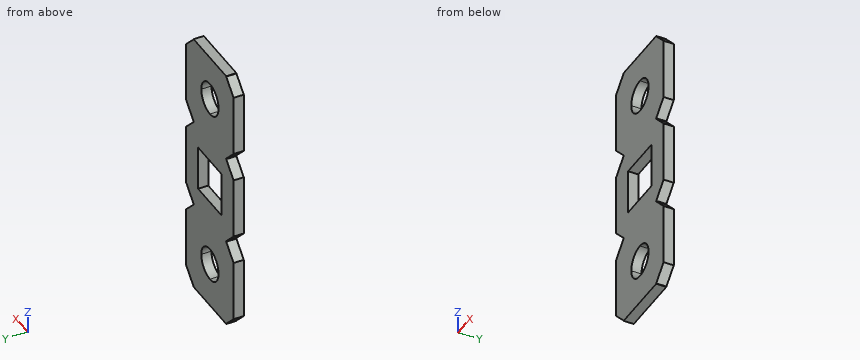
from build123d import *

# Parameters (mm, degrees)
STOCK_HS_LOCK_BAR_3_LONG_1_OUTLINE_W = 6.35
STOCK_HS_LOCK_BAR_3_LONG_1_OUTLINE_H = 6.35
STOCK_HS_LOCK_BAR_3_LONG_1_DEPTH     = 1.4224
BOSS_EXTRUDE1_START                  = -1.4224
BOSS_EXTRUDE1_DEPTH                  = 1.4224


# Read off the part's stored shape, not the designer's step: Stock-HS lock bar 3 long-1
with BuildPart() as part:
    # Stock-HS lock bar 3 long-1 outline → Stock-HS lock bar 3 long-1 (new body)
    with BuildSketch(Plane(origin=(0, 0, 0), x_dir=(1, 0, 0), z_dir=(0, 1, 0))):
        with BuildLine():
            Line((12.7, 36.073014945), (10.762817506, 38.010197439))
            ThreePointArc((10.762817506, 38.010197439), (10.725620068, 38.1), (10.762817506, 38.189802561))
            Line((10.762817506, 38.189802561), (12.7, 40.126985055))
            Line((12.7, 40.126985055), (12.7, 48.773014945))
            Line((12.7, 48.773014945), (10.762817506, 50.710197439))
            ThreePointArc((10.762817506, 50.710197439), (10.725620068, 50.8), (10.762817506, 50.889802561))
            Line((10.762817506, 50.889802561), (12.7, 52.826985055))
            Line((12.7, 52.826985055), (12.7, 61.473014945))
            Line((12.7, 61.473014945), (10.762817506, 63.410197439))
            ThreePointArc((10.762817506, 63.410197439), (10.735287367, 63.451399204), (10.725620068, 63.5))
            Line((10.725620068, 63.5), (1.974379932, 63.5))
            ThreePointArc((1.974379932, 63.5), (1.964712633, 63.451399204), (1.937182494, 63.410197439))
            Line((1.937182494, 63.410197439), (0, 61.473014945))
            Line((0, 61.473014945), (0, 52.826985055))
            Line((0, 52.826985055), (1.937182494, 50.889802561))
            ThreePointArc((1.937182494, 50.889802561), (1.974379932, 50.8), (1.937182494, 50.710197439))
            Line((1.937182494, 50.710197439), (0, 48.773014945))
            Line((0, 48.773014945), (0, 40.126985055))
            Line((0, 40.126985055), (1.937182494, 38.189802561))
            ThreePointArc((1.937182494, 38.189802561), (1.974379932, 38.1), (1.937182494, 38.010197439))
            Line((1.937182494, 38.010197439), (0, 36.073014945))
            Line((0, 36.073014945), (0, 27.426985055))
            Line((0, 27.426985055), (1.937182494, 25.489802561))
            ThreePointArc((1.937182494, 25.489802561), (1.964712633, 25.448600796), (1.974379932, 25.4))
            Line((1.974379932, 25.4), (10.725620068, 25.4))
            ThreePointArc((10.725620068, 25.4), (10.735287367, 25.448600796), (10.762817506, 25.489802561))
            Line((10.762817506, 25.489802561), (12.7, 27.426985055))
            Line((12.7, 27.426985055), (12.7, 36.073014945))
        make_face()
        with BuildLine():
            Line((4.0386, 29.9466), (4.0386, 33.5534))
            ThreePointArc((4.0386, 33.5534), (4.187389755, 33.912610245), (4.5466, 34.0614))
            Line((4.5466, 34.0614), (8.1534, 34.0614))
            ThreePointArc((8.1534, 34.0614), (8.512610245, 33.912610245), (8.6614, 33.5534))
            Line((8.6614, 33.5534), (8.6614, 29.9466))
            ThreePointArc((8.6614, 29.9466), (8.512610245, 29.587389755), (8.1534, 29.4386))
            Line((8.1534, 29.4386), (4.5466, 29.4386))
            ThreePointArc((4.5466, 29.4386), (4.187389755, 29.587389755), (4.0386, 29.9466))
        make_face(mode=Mode.SUBTRACT)
        with Locations((6.35, 44.45)):
            Rectangle(STOCK_HS_LOCK_BAR_3_LONG_1_OUTLINE_W, STOCK_HS_LOCK_BAR_3_LONG_1_OUTLINE_H, mode=Mode.SUBTRACT)
        with BuildLine():
            Line((4.0386, 55.3466), (4.0386, 58.9534))
            ThreePointArc((4.0386, 58.9534), (4.187389755, 59.312610245), (4.5466, 59.4614))
            Line((4.5466, 59.4614), (8.1534, 59.4614))
            ThreePointArc((8.1534, 59.4614), (8.512610245, 59.312610245), (8.6614, 58.9534))
            Line((8.6614, 58.9534), (8.6614, 55.3466))
            ThreePointArc((8.6614, 55.3466), (8.512610245, 54.987389755), (8.1534, 54.8386))
            Line((8.1534, 54.8386), (4.5466, 54.8386))
            ThreePointArc((4.5466, 54.8386), (4.187389755, 54.987389755), (4.0386, 55.3466))
        make_face(mode=Mode.SUBTRACT)
    extrude(amount=STOCK_HS_LOCK_BAR_3_LONG_1_DEPTH)

    # Sketch1 → Boss-Extrude1 (add)
    with BuildSketch(Plane(origin=(0, 1.4224, 0), x_dir=(1, 0, 0), z_dir=(0, 1, 0)).offset(BOSS_EXTRUDE1_START)):
        with BuildLine():
            Line((4.0386, 33.5534), (4.0386, 31.75))
            ThreePointArc((4.0386, 31.75), (4.715593386, 33.384406614), (6.35, 34.0614))
            Line((6.35, 34.0614), (4.5466, 34.0614))
            ThreePointArc((4.5466, 34.0614), (4.187389755, 33.912610245), (4.0386, 33.5534))
        make_face()
        with BuildLine():
            Line((8.1534, 34.0614), (6.35, 34.0614))
            ThreePointArc((6.35, 34.0614), (7.984406614, 33.384406614), (8.6614, 31.75))
            Line((8.6614, 31.75), (8.6614, 33.5534))
            ThreePointArc((8.6614, 33.5534), (8.512610245, 33.912610245), (8.1534, 34.0614))
        make_face()
        with BuildLine():
            ThreePointArc((8.6614, 31.75), (7.984406614, 30.115593386), (6.35, 29.4386))
            Line((6.35, 29.4386), (8.1534, 29.4386))
            ThreePointArc((8.1534, 29.4386), (8.512610245, 29.587389755), (8.6614, 29.9466))
            Line((8.6614, 29.9466), (8.6614, 31.75))
        make_face()
        with BuildLine():
            Line((4.0386, 31.75), (4.0386, 29.9466))
            ThreePointArc((4.0386, 29.9466), (4.187389755, 29.587389755), (4.5466, 29.4386))
            Line((4.5466, 29.4386), (6.35, 29.4386))
            ThreePointArc((6.35, 29.4386), (4.715593386, 30.115593386), (4.0386, 31.75))
        make_face()
        with BuildLine():
            ThreePointArc((8.6614, 57.15), (7.984406614, 55.515593386), (6.35, 54.8386))
            Line((6.35, 54.8386), (8.1534, 54.8386))
            ThreePointArc((8.1534, 54.8386), (8.512610245, 54.987389755), (8.6614, 55.3466))
            Line((8.6614, 55.3466), (8.6614, 57.15))
        make_face()
        with BuildLine():
            ThreePointArc((4.0386, 55.3466), (4.187389755, 54.987389755), (4.5466, 54.8386))
            Line((4.5466, 54.8386), (6.35, 54.8386))
            ThreePointArc((6.35, 54.8386), (4.715593386, 55.515593386), (4.0386, 57.15))
            Line((4.0386, 57.15), (4.0386, 55.3466))
        make_face()
        with BuildLine():
            ThreePointArc((6.350000002, 59.4614), (7.984406615, 58.784406613), (8.6614, 57.15))
            Line((8.6614, 57.15), (8.6614, 58.9534))
            ThreePointArc((8.6614, 58.9534), (8.512610245, 59.312610245), (8.1534, 59.4614))
            Line((8.1534, 59.4614), (6.350000002, 59.4614))
        make_face()
        with BuildLine():
            Line((4.0386, 58.9534), (4.0386, 57.15))
            ThreePointArc((4.0386, 57.15), (4.715593387, 58.784406615), (6.350000002, 59.4614))
            Line((6.350000002, 59.4614), (4.5466, 59.4614))
            ThreePointArc((4.5466, 59.4614), (4.187389755, 59.312610245), (4.0386, 58.9534))
        make_face()
    extrude(amount=BOSS_EXTRUDE1_DEPTH)


solid = part.part
Design review of the part built by this model. Coordinates are the model's own, in mm. Round coordinates to 2 decimals unless told otherwise and drop trailing zeros. Write each loop counter-clockwise with the first axis right and the second up, starting at its lowest first coordinate (ties: lowest second). Pieces come first, ordered by that corner, then holes.
Item 1: Wall thickness on L1, parallel to Z at x = 3.25, y = 0.7 (3 decimals); L2, parallel to X at y = 0.3, z = -44 (3 decimals); L3, parallel to Z at x = 8, y = 0.75 (3 decimals): over which ranges is each line inside the solid? List them lowest first.
Item 2: Consider section A-A on z = -45. Give the boundary of the cut face in (x, y) (3 decimals).
Item 3: Consider section B-B on x = 3.5. Give the boundary of the cut face in (y, z) (3 decimals), and give its area (3 significant figures).
Item 4: Consider section D-D on y = 0.3. Count the separate pieces of the cut face and the enclosed holes in it, and give its area (3 significant figures).
Item 5: Consider section C-C on x = 5. Give the boundary of the cut face in (y, z) (3 decimals), and give its area (3 significant figures).
Check values:
1. L1: z = -63.5 to -47.625, -41.275 to -25.4
1. L2: x = 0 to 3.175, 9.525 to 12.7
1. L3: z = -63.5 to -58.769, -55.531 to -47.625, -41.275 to -33.369, -30.131 to -25.4
2. outline: (0, 0) - (3.175, 0) - (3.175, 1.422) - (0, 1.422) - close; (9.525, 0) - (12.7, 0) - (12.7, 1.422) - (9.525, 1.422) - close
3. outline: (0, -63.5) - (1.422, -63.5) - (1.422, -47.625) - (0, -47.625) - close; (0, -41.275) - (1.422, -41.275) - (1.422, -25.4) - (0, -25.4) - close
3. area: 45.2 mm2
4. separate pieces: 1
4. enclosed holes: 3
4. area: 385 mm2
5. outline: (0, -63.5) - (1.422, -63.5) - (1.422, -59.026) - (0, -59.026) - close; (0, -55.274) - (1.422, -55.274) - (1.422, -47.625) - (0, -47.625) - close; (0, -41.275) - (1.422, -41.275) - (1.422, -33.626) - (0, -33.626) - close; (0, -29.874) - (1.422, -29.874) - (1.422, -25.4) - (0, -25.4) - close
5. area: 34.5 mm2
